Print and shaded views of the part. All mm, measured from the part's lowest x, y and z. A direction names the side the tool comes from. Coordinates: 2 decimals unless noted, no trailing zeros. Order: outer loops, then holes, each group sorted by start corner. A loop starts at its lowest first (then second) coordinate and runs counter-clockwise, first axis right, second up. Notation, with made-up numbers: M -31.75,87.25 L 0.25,87.25 A24 ccw 0.25,97.25 Z; hole C 36,42 d11. An arc over 180 degrees is marked long. One line per item, written item: value.
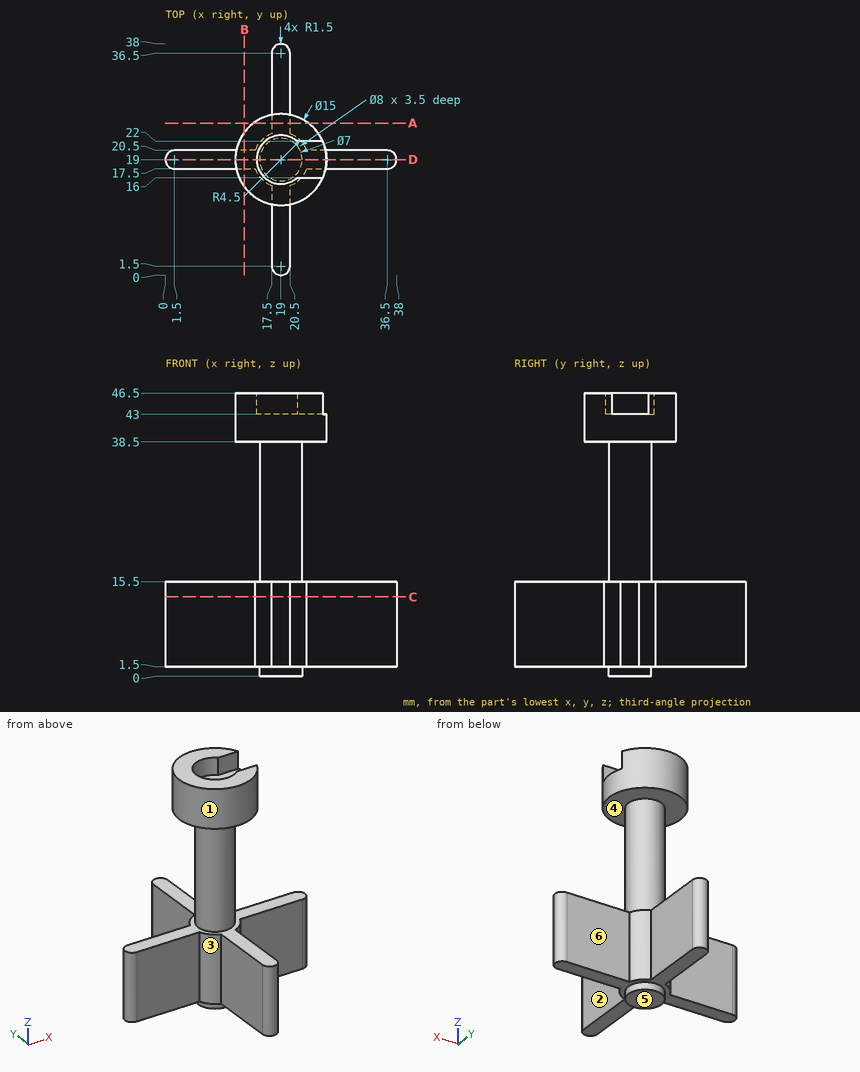
Q1. Slice it at A-A (y = 25). List the corners of the cut face in (x, z), plus the area to 3 significant figures.
Recorded:
outline: M 14.5,38.5 L 23.5,38.5 L 23.5,46.5 L 14.5,46.5 Z; M 17.5,1.5 L 20.5,1.5 L 20.5,15.5 L 17.5,15.5 Z
area: 114 mm^2
Q2. Which spindle directions (+Z, -Z, +X, -X, +Y, -Y) get a long thin tool onto all of the face, cutting with end or side? Do the marked faces 1, 2 and 3. Say none if no direction does.
Recorded:
face 1: +Z
face 2: -Z, +X, -Y
face 3: -Z, -X, -Y
Q3. Slice it at C-C (z = 13). List the corners of the cut face in (x, y).
Recorded:
outline: M 1.5,17.5 L 14.76,17.5 A4.5 ccw 17.5,14.76 L 17.5,1.5 A1.5 ccw 20.5,1.5 L 20.5,14.76 A4.5 ccw 23.24,17.5 L 36.5,17.5 A1.5 ccw 36.5,20.5 L 23.24,20.5 A4.5 ccw 20.5,23.24 L 20.5,36.5 A1.5 ccw 17.5,36.5 L 17.5,23.24 A4.5 ccw 14.76,20.5 L 1.5,20.5 A1.5 ccw Z
Q4. Drill centre lines: line 1 along Y through (x, z) = (19, 44); line 2 along Z through (x, y) = (12, 18.5); line 3 along Y through (x, z) = (2.5, 11). Where is each one in solid material? Low to high.
Recorded:
line 1: y = 11.5 to 15, 23 to 26.5
line 2: z = 1.5 to 15.5, 38.5 to 46.5
line 3: y = 17.5 to 20.5
Q5. Slice it at D-D (y = 19). List the corners of the cut face in (x, z), plus the area to 3 significant figures.
Recorded:
outline: M 0,1.5 L 15.5,1.5 L 15.5,0 L 22.5,0 L 22.5,1.5 L 38,1.5 L 38,15.5 L 22.5,15.5 L 22.5,38.5 L 26.5,38.5 L 26.5,43 L 15,43 L 15,46.5 L 11.5,46.5 L 11.5,38.5 L 15.5,38.5 L 15.5,15.5 L 0,15.5 Z
area: 783 mm^2
Q6. Pin check, flat tips, straight feed: pin 1 Ø4 at (x, z) = (7, 7) entering from -Y; pin 2 Ø4 at (x, z) = (24, 45) entering from +Y; pin 3 Ø6 at (x, z) = (15, 8.5) entering from -Y. Stop position of each tip, or through.
Recorded:
pin 1: stops at y = 17.5
pin 2: stops at y = 25.87
pin 3: stops at y = 0.38
Q7. Mould opens along Z. For the marked faces 4, 5 and 6 say: released by +Z, released by -Z, zero draft, split by the parting line, or undercut.
Recorded:
face 4: undercut
face 5: released by -Z
face 6: zero draft
